```python
from build123d import *

# Parameters (mm, degrees)
SKETCH1_R           = 1.6
SKETCH1_R_2         = 2.75
BOSS_EXTRUDE1_DEPTH = 2.5


with BuildPart() as part:
    # Sketch1 → Boss-Extrude1 (new body)
    with BuildSketch(Plane(origin=(0, 0, 0), x_dir=(1, 0, 0), z_dir=(0, 1, 0))):
        with BuildLine():
            Line((35.712808515, 6.287191485), (-35.712808515, 6.287191485))
            Line((-35.712808515, 6.287191485), (-35.712808515, 4.5))
            ThreePointArc((-35.712808515, 4.5), (-40.212808515, 0), (-35.712808515, -4.5))
            Line((-35.712808515, -4.5), (-35.712808515, -6.287191485))
            Line((-35.712808515, -6.287191485), (35.712808515, -6.287191485))
            Line((35.712808515, -6.287191485), (35.712808515, -4.5))
            ThreePointArc((35.712808515, -4.5), (40.212808515, 0), (35.712808515, 4.5))
            Line((35.712808515, 4.5), (35.712808515, 6.287191485))
        make_face()
        with Locations(Location((35.712808515, 0, 0), (0, 0, 270))):
            Circle(SKETCH1_R, mode=Mode.SUBTRACT)
        with Locations(Location((0, 0, 0), (0, 0, 270))):
            Circle(SKETCH1_R_2, mode=Mode.SUBTRACT)
        with Locations(Location((-35.712808515, 0, 0), (0, 0, 270))):
            Circle(SKETCH1_R, mode=Mode.SUBTRACT)
    extrude(amount=BOSS_EXTRUDE1_DEPTH)


solid = part.part
```
Could you check a few things on this model? Use its own coordinates, in mm. A direction names the side the tool comes from. Coordinates: 2 decimals unless noted, no trailing zeros. Order: outer loops, then holes, each group sorted by start corner. A loop starts at its lowest first (then second) coordinate and runs counter-clockwise, first axis right, second up. Notation, with made-up numbers: M 88,29.25 L 112,29.25 A25 cw 112,63.25 Z; hole C 53,65.5 d7. An arc over 180 degrees is marked long. Use a Markdown table: item, result. Add a question column.
Q1. If I drill on L1, parallel to X at y = 0.6, z = 0; L2, parallel to X at y = 2, z = -5; L3, parallel to X at y = 0.4, z = -0.5, over which ranges is the centre line in solid material (lowest first)?
Q2. I want a section at A-A on z = 0. List the corners of the cut face in (x, y) for me, then the cut area to 3 significant figures.
Q3. I want a section at C-C on x = 0. List the corners of the cut face in (y, z) for me.
Q4. I want a section at B-B on y = 1.5. List the corners of the cut face in (x, z) for me.
Q5. Which directions (+Z, -Z, +X, -X, +Y, -Y) give clear straight access to the entire face, cutting with the end or side of a thin tool? Please do faces 4 (the cylindrical face through (-2.685, 1.232, -0.596)), 5 (the flat face through (35.713, 1, -5)), 6 (the cylindrical face through (40.21, 1.23, 0.1)), 7 (the flat face through (-35.713, 1, -5)), 8 (the flat face through (35.713, 1, 5)).
Q6. We'd pull the mould along Z, two halves only. Please class faces 1 (the cylindrical face through (34.293, 1.232, 0.738)), 2 (the flat face through (0, 1, 6.287)), 3 (the flat face through (-35.713, 1, 5)): pulls with the +Z half, pulls with the -Z half, needs draft (parallel to the pull), parting line crosses it, or undercut.
Q7. I'm going to push flat-ended pins straight in: pin 1 (1.4 mm diameter, centred on y = 1.5, z = 5.5, fed in from -X); pin 2 (0.5 mm diameter, centred on y = 0.5, z = -5, fed in from +X). Where does each tip first touch, or does it pass through?
Checked values:
| question | item | result |
|---|---|---|
| 1 | L1 | -40.21 to -37.31, -34.11 to -2.75, 2.75 to 34.11, 37.31 to 40.21 |
| 1 | L2 | -35.71 to 35.71 |
| 1 | L3 | -40.18 to -37.23, -34.19 to -2.7, 2.7 to 34.19, 37.23 to 40.18 |
| 2 | outline | M -40.21,0 L -37.31,0 L -37.31,2.5 L -40.21,2.5 Z; M -34.11,0 L -2.75,0 L -2.75,2.5 L -34.11,2.5 Z; M 2.75,0 L 34.11,0 L 34.11,2.5 L 2.75,2.5 Z; M 37.31,0 L 40.21,0 L 40.21,2.5 L 37.31,2.5 Z |
| 2 | area | 171 mm² |
| 3 | outline | M 0,-6.29 L 2.5,-6.29 L 2.5,-2.75 L 0,-2.75 Z; M 0,2.75 L 2.5,2.75 L 2.5,6.29 L 0,6.29 Z |
| 4 | outline | M -35.71,-6.29 L 35.71,-6.29 L 35.71,-4.5 A4.5 ccw 35.71,4.5 L 35.71,6.29 L -35.71,6.29 L -35.71,4.5 A4.5 ccw -35.71,-4.5 Z; hole C -35.71,0 d3.2; hole C 0,0 d5.5; hole C 35.71,0 d3.2 |
| 5 | face 4 | +Y, -Y |
| 5 | face 5 | -Z, +X, +Y, -Y |
| 5 | face 6 | +X, +Y, -Y |
| 5 | face 7 | -Z, -X, +Y, -Y |
| 5 | face 8 | +Z, +X, +Y, -Y |
| 6 | face 1 | undercut |
| 6 | face 2 | pulls with the +Z half |
| 6 | face 3 | needs draft |
| 7 | pin 1 | x = -35.71 |
| 7 | pin 2 | x = 35.71 |
